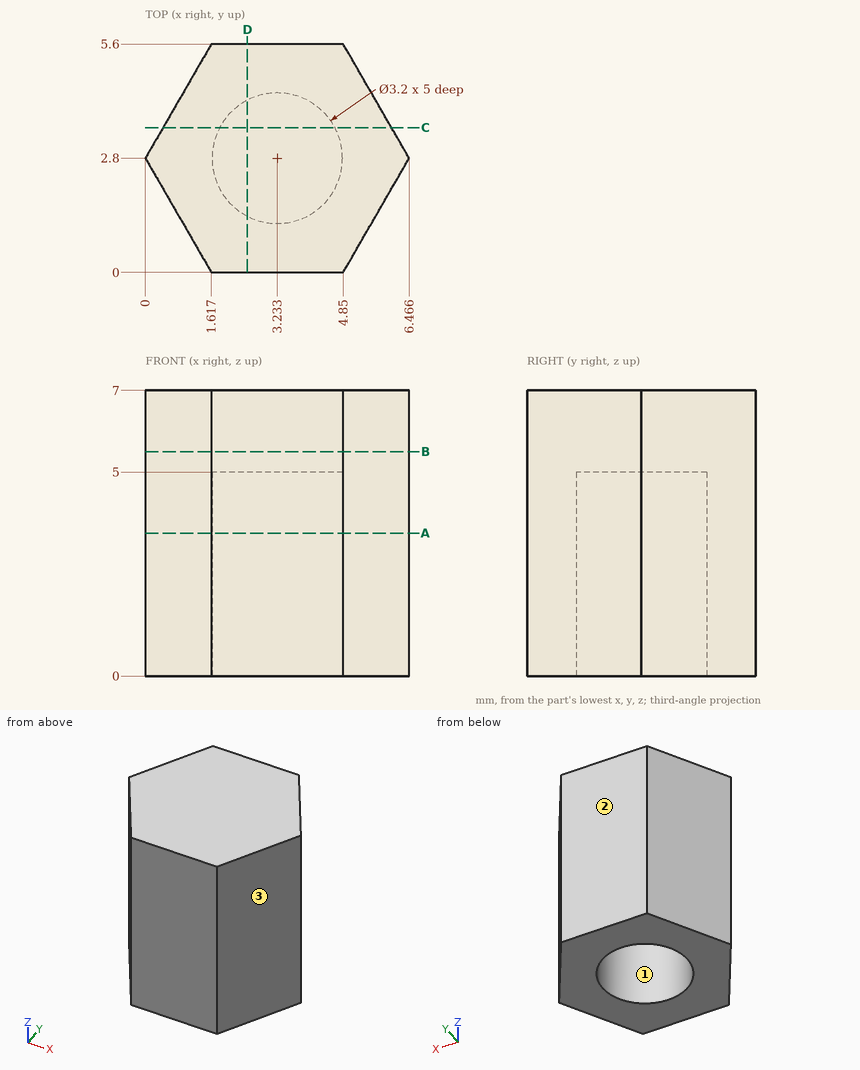
The figure shows three views and two pictorial views of one solid part (mm, origin at its lowest corner). Answer the questions. Round coordinates to 2 decimals unless told otherwise and drop trailing zeros. Loops run counter-clockwise (first coordinate to the right, second up) from the corner with the lowest first, then second, coordinate; pieces in that order, holes last. Notation, with made-up numbers: M 70.5,-23 L 111.5,-23 A27 cw 111.5,11 Z; hole C 20.25,-16.75 d11. An arc over 180 degrees is marked long. Return JSON: item names as keys, results as strings.
Q1. Find section B-B, the plane z = 5.5. Determine the outline of the cut face in (x, y).
Results list:
{"outline": "M 0,2.8 L 1.62,0 L 4.85,0 L 6.47,2.8 L 4.85,5.6 L 1.62,5.6 Z"}
Q2. Find the intervals of material crossed by line 1 along Y through (x, z) = (3.25, 3.5); line 2 along Y through (x, z) = (2.75, 1.5) (1 decimal); line 3 along Y through (x, z) = (5.25, 5.5) (1 decimal), in increasing order. Write a range as from..to.
Results list:
{"line 1": "y = 0..1.2, 4.4..5.6", "line 2": "y = 0..1.3, 4.3..5.6", "line 3": "y = 0.7..4.9"}
Q3. Find section A-A, the plane z = 3.5. Determine the outline of the cut face in (x, y), plus the area to 3 significant figures.
Results list:
{"outline": "M 0,2.8 L 1.62,0 L 4.85,0 L 6.47,2.8 L 4.85,5.6 L 1.62,5.6 Z; hole C 3.23,2.8 d3.2", "area": "19.1 mm2"}
Q4. The mould has two halves that part along X. Classify the marked faces 1, 2 and 3: released by +X, released by -X, zero draft, split by the parting line, or undercut.
Results list:
{"face 1": "undercut", "face 2": "zero draft", "face 3": "released by +X"}
Q5. Find section C-C, the plane y = 3.55. Determine the outline of the cut face in (x, z).
Results list:
{"outline": "M 0.43,0 L 1.82,0 L 1.82,5 L 4.65,5 L 4.65,0 L 6.03,0 L 6.03,7 L 0.43,7 Z"}
Q6. Each of these flat-tipped pins is pushed along its axis until it touches: pin 1 Ø3 at (x, y) = (3.23, 2.8) entering from -Z; pin 2 Ø1 at (y, z) = (2, 3) entering from -X. Where does it stop, or does it pass through?
Results list:
{"pin 1": "stops at z = 5", "pin 2": "stops at x = 0.17"}
Q7. Find section D-D, the plane x = 2.5. Determine the outline of the cut face in (y, z).
Results list:
{"outline": "M 0,0 L 1.38,0 L 1.38,5 L 4.22,5 L 4.22,0 L 5.6,0 L 5.6,7 L 0,7 Z"}
